Check sheet for the drawn part. Datum: minimum x, y, z corner. Units: mm. A direction names the side the tool comes from. Give positions to 0.01 mm unless a question says otherwise; leave off trailing zeros. Write each loop counter-clockwise with the first axis right and the second up, starting at its lowest first coordinate (ties: lowest second). Pieces come first, ordered by that corner, then holes. Notation, with made-up numbers: (-19, -22.75) - (20, -22.75) arc R27 cw to (20, 9.25) - close; hole circle Ø3 at (4, 21). An arc over 180 degrees is marked (long way). Answer as a JSON object with one key per item and string values. Group by question number.
Item 1: Go/stop test with flat-tipped pins: pin 1 (12.5 mm diameter, centred on x = 23.5, z = 249, fed in from +Y); pin 2 (12 mm diameter, centred on x = 9.5, y = 40, fed in from -Z). Record where each tip stops, or that it passes through.
Item 2: Scan lines: line 1 along Y through (x, z) = (14.5, 79.5); line 2 along Z through (x, y) = (6.5, 25). Record each from-to range of solid material in increasing order. Write a range as [from, to].
Item 3: Tool access check on the marked faces 1 and 2. Record the directions out of +Z, -Z, +X, -X, +Y, -Y that give a thin tool (end or side, any length) a straight path to the whole face; none if there is none.
Item 4: Sectioned sample at A-A, the plane y = 27. Record the boundary of the cut face in (x, z), and give its area (3 significant figures).
Item 5: Sectioned sample at B-B, the plane z = 157. Record the boundary of the cut face in (x, y), and give its area (3 significant figures).
Item 6: Sectioned sample at C-C, the plane x = 14. Record the boundary of the cut face in (y, z).
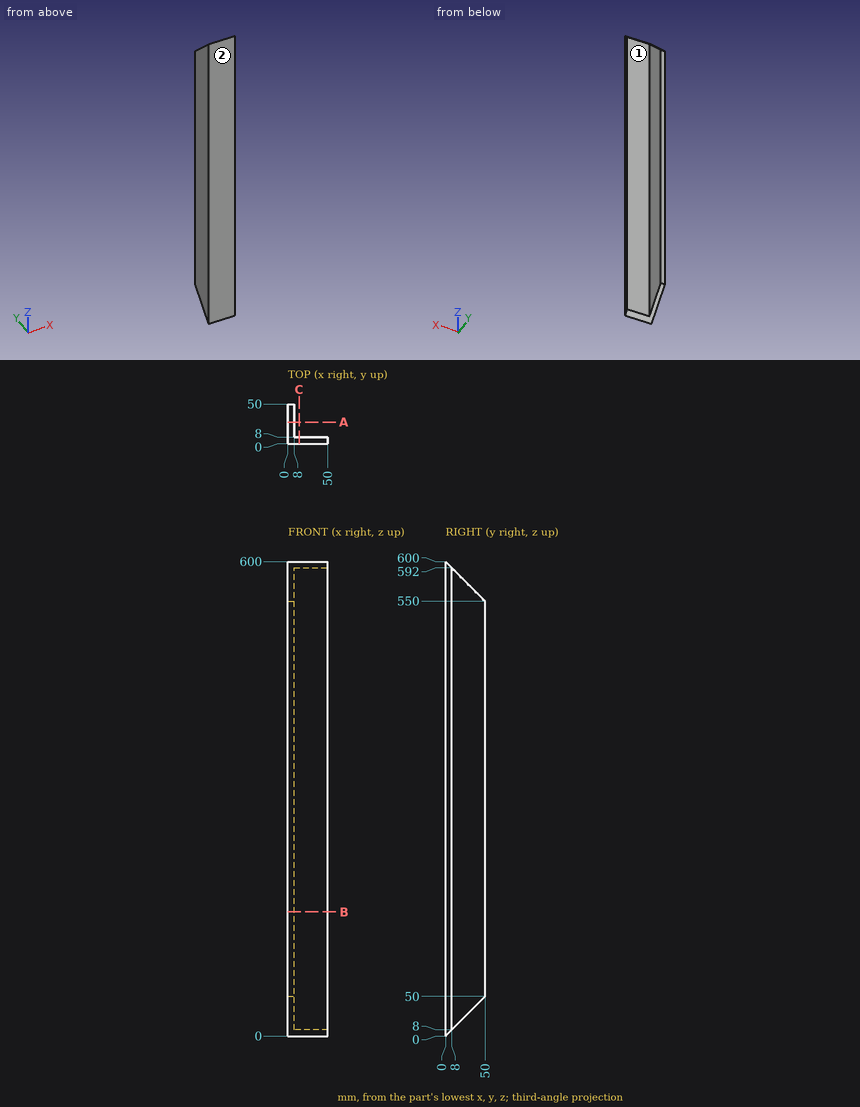
Geometry check:
{
 "1": {"pin 1": "y = 8", "pin 2": "z = 34.19"},
 "2": {"line 1": "[0, 8]", "line 2": "[25, 575]"},
 "3": {"face 1": "+Z, -Z, +X, +Y", "face 2": "+Z, -Z, +X, -X, -Y"},
 "4": {"outline": "(0, 27) - (8, 27) - (8, 573) - (0, 573) - close", "area": "4,370 mm^2"},
 "5": {"outline": "(0, 0) - (50, 0) - (50, 8) - (8, 8) - (8, 50) - (0, 50) - close", "area": "736 mm^2"},
 "6": {"outline": "(0, 0) - (8, 8) - (8, 592) - (0, 600) - close"}
}
